```python
from build123d import *

# Parameters (mm, degrees)
SKETCH1_W           = 500
SKETCH1_H           = 500
SKETCH1_R           = 100
BOSS_EXTRUDE1_DEPTH = 2
SKETCH_1_R          = 3.25
CUT_EXTRUDE_1_DEPTH = 10


with BuildPart() as part:
    # Sketch1 → Boss-Extrude1 (new body)
    with BuildSketch(Plane(origin=(0, 0, 0), x_dir=(1, 0, 0), z_dir=(0, 1, 0))):
        with Locations((250, 250)):
            Rectangle(SKETCH1_W, SKETCH1_H)
        with Locations(Location((250, 250, 0), (0, 0, 270))):
            Circle(SKETCH1_R, mode=Mode.SUBTRACT)
    extrude(amount=BOSS_EXTRUDE1_DEPTH)

    # 草图1 → 切除-拉伸1 (cut)
    with BuildSketch(Plane(origin=(0, 2, 0), x_dir=(1, 0, 0), z_dir=(0, 1, 0))):
        with Locations(Location((245.5, 33.4, 0), (0, 0, 270))):
            Circle(SKETCH_1_R)
        with Locations(Location((33.4, 250.5, 0), (0, 0, 270))):
            Circle(SKETCH_1_R)
        with Locations(Location((462.6, 245.5, 0), (0, 0, 270))):
            Circle(SKETCH_1_R)
        with Locations(Location((250.5, 462.6, 0), (0, 0, 270))):
            Circle(SKETCH_1_R)
    extrude(amount=-CUT_EXTRUDE_1_DEPTH, mode=Mode.SUBTRACT)


solid = part.part
```
Build history of the part. All positions in model axes, mm. Round coordinates to 2 decimals unless told otherwise and drop trailing zeros. Write each loop counter-clockwise with the first axis right and the second up, starting at its lowest first coordinate (ties: lowest second). Pieces come first, ordered by that corner, then holes.
1) Band-saw the part on A-A, the plane z = -286.5. List the corners of the cut face in (x, y).
2) Band-saw the part on B-B, the plane y = 1.2. List the corners of the cut face in (x, z).
3) Drill centre lines: probe 1 along X at (y, z) = (1.3, -245.5); probe 2 along Z at (x, y) = (250.5, 1.2); probe 3 along X at (y, z) = (0.55, -250). Where is each one in solid material? Low to high.
4) Band-saw the part on C-C, the plane x = 324. List the corners of the cut face in (y, z).
5) Mould opens along X. For faces 1 (the flat face through (247, 0, -365)), 2 (the cylindrical face through (254.397, 0.986, -349.903)) say: +X half, -X half, draft (parallel to the pull), parting line (faces both ways), or undercut.
6) Pin check, flat tip, straight feed: pin 1 (2 mm diameter, centred on x = 422.5, z = -100.5, fed in from -Y). Stop position of the tip, or through.
Ans:
1. outline: (0, 0) - (156.9, 0) - (156.9, 2) - (0, 2) - close; (343.1, 0) - (500, 0) - (500, 2) - (343.1, 2) - close
2. outline: (0, -500) - (500, -500) - (500, 0) - (0, 0) - close; hole circle Ø6.5 at (33.4, -250.5); hole circle Ø200 at (250, -250); hole circle Ø6.5 at (245.5, -33.4); hole circle Ø6.5 at (250.5, -462.6); hole circle Ø6.5 at (462.6, -245.5)
3. probe 1: x = 0 to 150.1, 349.9 to 459.35, 465.85 to 500
3. probe 2: z = -500 to -465.85, -459.35 to -350, -150 to 0
3. probe 3: x = 0 to 30.19, 36.61 to 150, 350 to 500
4. outline: (0, -500) - (2, -500) - (2, -317.26) - (0, -317.26) - close; (0, -182.74) - (2, -182.74) - (2, 0) - (0, 0) - close
5. face 1: draft
5. face 2: undercut
6. pin 1: stops at y = 0
